Design review of the part built by this model. Coordinates are the model's own, in mm. Give positions to 0.01 mm unless a question says otherwise; leave off trailing zeros. Loops run counter-clockwise (first coordinate to the right, second up) from the corner with the lowest first, then second, coordinate; pieces in that order, holes last. Notation, with made-up numbers: (-12, 63) -> (31, 63) arc R15 cw to (31, 92) -> close; hole circle Ø1 at (-12.75, -34). An arc over 180 degrees is marked (long way). Use a Markdown table: item, result. Add a question column.
1. Add section B-B (y = 0). State the section outline as (x, z) points.
2. Add section C-C (z = 4.75). State the section outline as (x, y) points, and give its area (3 significant figures).
3. Add section A-A (x = 0). State the section outline as (y, z) points.
4. For pin 1 Ø9.5 at (x, y) = (2.5, 0) entering from +Z; pin 2 Ø6.5 at (x, y) = (0, 0) entering from +Z, all flat-tipped, find the tip position at first contact; note any pin that passes through.
5. Add section D-D (x = -6). State the section outline as (y, z) points.
6. To check wall thickness, follow line 1 (Y direction, x = 0, z = -2.1); line 2 (Y direction, x = 0, z = 3.85); line 3 (Z direction, x = 1.75, y = -5.5). State the ranges of each line that lie inside material, in increasing order.
7. Draft analysis for pull direction Y (two halves, no side actions). For faces 1 (the cylindrical face through (4.38, -8.43, 2.96)), 2 (the flat face through (-13.5, 9, 2)), 3 (the flat face through (0, -13.5, 2)), 4 (the flat face through (2, -4, 0)), state which applies: pulls with the +Y half, pulls with the -Y half, needs draft (parallel to the pull), parting line crosses it, or undercut.
```python
from build123d import *

# Parameters (mm, degrees)
F0_W     = 27
F0_H     = 45.5
F0_R     = 9.5
F1_DEPTH = 6
F0_R_2   = 4
F2_DEPTH = 3


with BuildPart() as f1:
    # F0 (on Top) → F1 (new body)
    with BuildSketch(Plane.XY):
        with Locations((0, 9.25)):
            Rectangle(F0_W, F0_H)
        Circle(F0_R, mode=Mode.SUBTRACT)
    extrude(amount=F1_DEPTH)

    # F0 (on Top) → F2 (join)
    with BuildSketch(Plane.XY):
        with Locations((0, 9.25)):
            Rectangle(F0_W, F0_H)
        Circle(F0_R, mode=Mode.SUBTRACT)
        Circle(F0_R)
        Circle(F0_R_2, mode=Mode.SUBTRACT)
    extrude(amount=-F2_DEPTH)


solid = f1.part
```
Taken from the geometry:
| question | item | result |
|---|---|---|
| 1 | outline | (-13.5, -3) -> (-4, -3) -> (-4, 0) -> (-9.5, 0) -> (-9.5, 6) -> (-13.5, 6) -> close; (4, -3) -> (13.5, -3) -> (13.5, 6) -> (9.5, 6) -> (9.5, 0) -> (4, 0) -> close |
| 2 | outline | (-13.5, -13.5) -> (13.5, -13.5) -> (13.5, 32) -> (-13.5, 32) -> close; hole circle Ø19 at (0, 0) |
| 2 | area | 945 mm^2 |
| 3 | outline | (-13.5, -3) -> (-4, -3) -> (-4, 0) -> (-9.5, 0) -> (-9.5, 6) -> (-13.5, 6) -> close; (4, -3) -> (32, -3) -> (32, 6) -> (9.5, 6) -> (9.5, 0) -> (4, 0) -> close |
| 4 | pin 1 | stops at z = 0 |
| 4 | pin 2 | passes through |
| 5 | outline | (-13.5, -3) -> (32, -3) -> (32, 6) -> (7.37, 6) -> (7.37, 0) -> (-7.37, 0) -> (-7.37, 6) -> (-13.5, 6) -> close |
| 6 | line 1 | y = -13.5 to -4, 4 to 32 |
| 6 | line 2 | y = -13.5 to -9.5, 9.5 to 32 |
| 6 | line 3 | z = -3 to 0 |
| 7 | face 1 | undercut |
| 7 | face 2 | needs draft |
| 7 | face 3 | pulls with the -Y half |
| 7 | face 4 | undercut |
